from build123d import *

# Parameters (mm, degrees)
SKETCH1_R               = 6
SKETCH1_R_2             = 1.525
BOSS_EXTRUDE1_DEPTH     = 5
CUT_EXTRUDE1_DEPTH      = 198.040604952
CUT_EXTRUDE1_DEPTH_BACK = 198.040604952
SKETCH2_R               = 18.5


with BuildPart() as part:
    # Sketch1 → Boss-Extrude1 (new body)
    with BuildSketch(Plane(origin=(0, 0, 0), x_dir=(1, 0, 0), z_dir=(0, 1, 0))):
        Polygon((0, -40.379460215), (80, -40.467284232), (80, -180), (0, -180), align=None)
        with Locations(Location((40, -131.25, 0), (0, 0, 270))):
            Circle(SKETCH1_R, mode=Mode.SUBTRACT)
        with Locations(Location((24.5, -138.25, 0), (0, 0, 270))):
            Circle(SKETCH1_R_2, mode=Mode.SUBTRACT)
        with Locations(Location((55.5, -138.25, 0), (0, 0, 270))):
            Circle(SKETCH1_R_2, mode=Mode.SUBTRACT)
        with Locations(Location((32.25, -124.826606241, 0), (0, 0, 270))):
            Circle(SKETCH1_R_2, mode=Mode.SUBTRACT)
        with Locations(Location((47.75, -124.826606241, 0), (0, 0, 270))):
            Circle(SKETCH1_R_2, mode=Mode.SUBTRACT)
    extrude(amount=BOSS_EXTRUDE1_DEPTH)

    # Sketch2 → Cut-Extrude1 (cut, two sides: drawn at the far end of the back side and taken through both)
    with BuildSketch(Plane(origin=(0, 5, 0), x_dir=(1, 0, 0), z_dir=(0, 1, 0)).offset(-CUT_EXTRUDE1_DEPTH_BACK)):
        with Locations(Location((40, -138.25, 0), (0, 0, 270))):
            Circle(SKETCH2_R)
    extrude(amount=CUT_EXTRUDE1_DEPTH + CUT_EXTRUDE1_DEPTH_BACK, mode=Mode.SUBTRACT)


solid = part.part
Geometry: final body of the model. Coordinates: model frame, mm. Round coordinates to 2 decimals unless told otherwise and drop trailing zeros. Loops run counter-clockwise (first coordinate to the right, second up) from the corner with the lowest first, then second, coordinate; pieces in that order, holes last. Notation, with made-up numbers: M -15.75,16 L 10.25,16 A31 ccw 10.25,55 Z; hole C 75,58 d8. An arc over 180 degrees is marked long. Put each result on its own line as item: value. Start each with the question number.
(1) Contact query for flat-ended pins moving along their axis: pin 1 Ø4 at (x, z) = (19, 81) entering from -Y; pin 2 Ø2 at (x, y) = (55.5, 2) entering from -Z. Output: stop coordinate, or through.
(2) Section query B-B (x = 40). Return loops of the section in (y, z), then the cut area to 3 significant figures.
(3) Material intervals for line 1 along X through (y, z) = (3.9, 138.25); line 2 along Z through (x, y) = (60.5, 2.65); line 3 along Z through (x, y) = (42.5, 0.2), sorted ascending. Write a range as [from, to].
(4) Section query A-A (z = 138.25). Return loops of the section in (x, y).
(5) Draft query along X for faces 1 (the face through (80, 2, 109)), 2 (the face through (41, 5, 109)), 3 (the face through (45.557, 2.465, 155.896)), 4 (the face through (0, 2, 111)). Return one class per face: +X half, -X half, draft (parallel to the pull), parting line (faces both ways), or undercut.
(6) Section query C-C (y = 1.85). Return loops of the section in (x, z), then the cut area to 3 significant figures.
Findings below:
1. pin 1: stops at y = 0
1. pin 2: stops at z = 40.44
2. outline: M 0,40.42 L 5,40.42 L 5,119.75 L 0,119.75 Z; M 0,156.75 L 5,156.75 L 5,180 L 0,180 Z
2. area: 513 mm2
3. line 1: x = [0, 21.5], [58.5, 80]
3. line 2: z = [40.45, 180]
3. line 3: z = [40.43, 119.92], [156.58, 180]
4. outline: M 0,0 L 21.5,0 L 21.5,5 L 0,5 Z; M 58.5,0 L 80,0 L 80,5 L 58.5,5 Z
5. face 1: +X half
5. face 2: draft
5. face 3: undercut
5. face 4: -X half
6. outline: M 0,40.38 L 80,40.47 L 80,180 L 0,180 Z; hole C 40,138.25 d37
6. area: 10,100 mm2
